Part model, mm, in its own coordinate system. Face numbers are marked on the shaded views. A direction names the side the tool comes from. Round coordinates to 2 decimals unless told otherwise and drop trailing zeros. Loops run counter-clockwise (first coordinate to the right, second up) from the corner with the lowest first, then second, coordinate; pieces in that order, holes last.
(1) Mould opens along Z. For the marked faces 4, 5 and 6 say: +Z half, -Z half, draft (parallel to the pull), parting line (faces both ways), or undercut.
(2) Cut at B-B on x = -4.5. List the corners of the cut face in (y, z) (1 decimal), then the cut area to 3 significant figures.
(3) Tool access for the marked faces 1, 2 and 3: list every direction of +Z, -Z, +X, -X, +Y, -Y with a clear straight run to the whole face (end or side of a thin tool).
(4) Flat gauge pins, fed straight in: pin 1 (1 mm diameter, centred on x = 13.5, y = 3.5, fed in from -Z); pin 2 (3 mm diameter, centred on x = 5.5, z = 3, fed in from +Y); pin 3 (3 mm diameter, centred on y = 0.5, z = 6, fed in from +X). Where does each tip first touch, or does it go through?
(5) Cut at C-C on x = 10.5. List the corners of the cut face in (y, z), then the cut area to 3 significant figures.
(6) Cut at A-A on y = 0. List the corners of the cut face in (x, z) (3 decimals).
(7) Probe probe 1 along X at (y, z) = (-4.75, -4.25); probe 2 along Y at (x, z) = (15, 2.5); probe 3 along X at (y, z) = (-0.5, 1). List the from-to ranges inside material, lowest first.
Autodesk Inventor part; units mm, degrees
ref_plane "IP1_XY" through (0, 0, 0) normal (1, 0, 0) x (0, 0, -1)
ref_plane "IP1_YZ" through (0, 0, 0) normal (0, 0, -1) x (0, 1, 0)
ref_plane "IP1_ZX" through (0, 0, 0) normal (0, 1, 0) x (1, 0, 0)
sketch "Skizze_2" plane through (0, 0, 0) normal (0, 0, 1) x (1, 0, 0)
  line L0 (38, 0) -> (-10, 0)
  line L1 (-10, 0) -> (-10, 7)
  arc A0 (-9, 8) -> (-10, 7) centre (-9, 7) ccw
  line L2 (-9, 8) -> (0, 8)
  line L3 (0, 8) -> (0, 5.6)
  arc A1 (0, 5.6) -> (0.2772, 5.2193) centre (0.4, 5.6) ccw
  line L4 (0.2772, 5.2193) -> (0.8972, 5.0193)
  arc A2 (0.8972, 5.0193) -> (1.02, 5) centre (1.02, 5.4) ccw
  line L5 (1.02, 5) -> (34.08, 5)
  line L6 (34.08, 5) -> (35, 4.08)
  line L7 (35, 4.08) -> (35, 0)
  line L8 (35, 0) -> (-10, 0)
revolve "Revolution1" add sketch "Skizze_2" angle 360 about axis through (38, 0, 0) along (1, 0, 0)
thread "Thread1"
sketch "Skizze_1" plane through (-4.001, 0, 0) normal (1, 0, 0) x (0, 0, -1)
  line L0 (-3.995, -2.3065) -> (0, -4.613)
  line L1 (0, -4.613) -> (3.995, -2.3065)
  line L2 (3.995, -2.3065) -> (3.995, 2.3065)
  line L3 (3.995, 2.3065) -> (0, 4.613)
  line L4 (0, 4.613) -> (-3.995, 2.3065)
  line L5 (-3.995, 2.3065) -> (-3.995, -2.3065)
extrude "Extrusion1" cut sketch "Skizze_1" against normal blind 10.01
ref_plane "IP1_XY" through (0, 0, 0) normal (1, 0, 0) x (0, 0, -1)
ref_plane "IP1_YZ" through (0, 0, 0) normal (0, 0, -1) x (0, 1, 0)
ref_plane "IP1_ZX" through (0, 0, 0) normal (0, 1, 0) x (1, 0, 0)
ref_plane "IP2_XY" through (-10, 0, 0) normal (1, 0, 0) x (0, 0, -1)
ref_plane "IP2_YZ" through (-10, 0, 0) normal (0, 0, -1) x (0, 1, 0)
ref_plane "IP2_ZX" through (-10, 0, 0) normal (0, 1, 0) x (1, 0, 0)
ref_plane "IP3_XY" through (35, 0, 0) normal (1, 0, 0) x (0, 0, -1)
ref_plane "IP3_YZ" through (35, 0, 0) normal (0, 0, -1) x (0, 1, 0)
ref_plane "IP3_ZX" through (35, 0, 0) normal (0, 1, 0) x (1, 0, 0)
properties part number "Slotted head cap screw ISO 4762 - M10x35"
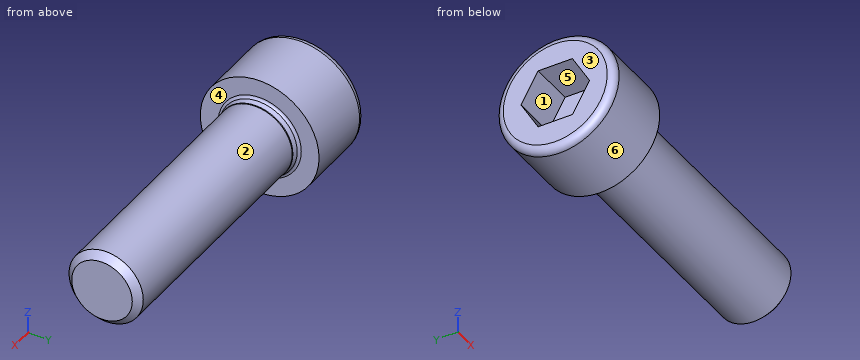
Final values:
1. face 4: draft
1. face 5: undercut
1. face 6: parting line
2. outline: circle Ø16 at (0, 0); hole (-4.6, 0) - (-2.3, -4) - (2.3, -4) - (4.6, 0) - (2.3, 4) - (-2.3, 4) - close
2. area: 146 mm2
3. face 1: -X
3. face 2: +X
3. face 3: +Z, -Z, -X, +Y, -Y
4. pin 1: stops at z = -4
4. pin 2: stops at y = 4.77
4. pin 3: stops at x = 34.56
5. outline: circle Ø10 at (0, 0)
5. area: 78.5 mm2
6. outline: (-10, -7) arc R1 ccw to (-9, -8) - (0, -8) - (0, -5.6) arc R0.4 cw to (0.277, -5.219) - (0.897, -5.019) arc R0.399 cw to (1.02, -5) - (34.08, -5) - (35, -4.08) - (35, 4.08) - (34.08, 5) - (1.02, 5) arc R0.399 cw to (0.897, 5.019) - (0.277, 5.219) arc R0.4 cw to (0, 5.6) - (0, 8) - (-9, 8) arc R1 ccw to (-10, 7) - (-10, 3.995) - (-4.001, 3.995) - (-4.001, -3.995) - (-10, -3.995) - close
7. probe 1: x = -10 to 0
7. probe 2: y = -4.33 to 4.33
7. probe 3: x = -4 to 35
